Autodesk Inventor part; units mm, degrees
ref_plane "YZ Plane" through (0, 0, 0) normal (1, 0, 0) x (0, 1, 0)
ref_plane "XZ Plane" through (0, 0, 0) normal (0, 1, 0) x (-1, 0, 0)
ref_plane "XY Plane" through (0, 0, 0) normal (0, 0, 1) x (1, 0, 0)
sketch "Sketch1" plane through (0, 0, 0) normal (0, 1, 0) x (-1, 0, 0)
  line L0 (0, 0) -> (90, 0)
  line L1 (90, 0) -> (90, -50)
  line L2 (90, -50) -> (0, -50)
  line L3 (0, -50) -> (0, 0)
  line L4 (0, 0) -> (0, -16.6667)
  line L5 (0, -16.6667) -> (6, -16.6667)
  dimension "d0" = 90
  dimension "d1" = 50
  dimension "d2" = 16.6667
  dimension "d3" = 6
extrude "Extrusion1" add sketch "Sketch1" along normal blind 6
sketch "Sketch3" plane through (0, 6, 0) normal (0, 1, 0) x (1, 0, 0)
  circle A0 centre (-13, 12.5) radius 2.75
  line L0 (0, 0) -> (0, 50)
  line L1 (-90, 0) -> (0, 0)
  circle A1 centre (-13, 37.5) radius 2.75
  line L2 (-13, 12.5) -> (-18, 12.5)
  line L3 (-23, 12.5) -> (-13, 12.5) construction
  line L4 (-23, 9.75) -> (-13, 9.75)
  line L5 (-13, 15.25) -> (-23, 15.25)
  arc A2 (-23, 15.25) -> (-23, 9.75) centre (-23, 12.5) ccw
  arc A3 (-13, 9.75) -> (-13, 15.25) centre (-13, 12.5) ccw
  line L6 (-13, 37.5) -> (-18, 37.5)
  line L7 (-13, 37.5) -> (-8, 37.5) construction
  line L8 (-23, 37.5) -> (-13, 37.5) construction
  line L9 (-23, 34.75) -> (-13, 34.75)
  line L10 (-13, 40.25) -> (-23, 40.25)
  arc A4 (-23, 40.25) -> (-23, 34.75) centre (-23, 37.5) ccw
  arc A5 (-13, 34.75) -> (-13, 40.25) centre (-13, 37.5) ccw
  dimension "d21" = 5.5
  dimension "d22" = 13
  dimension "d23" = 12.5
  dimension "d26" = 25
  dimension "d87" = 5
  dimension "d88" = 5
  dimension "d89" = 180
extrude "Extrusion3" cut sketch "Sketch3" against normal through all
sketch "Sketch4" plane through (0, 6, 0) normal (0, 1, 0) x (1, 0, 0)
  arc A0 (-13, 9.75) -> (-13, 15.25) centre (-13, 12.5) ccw
  line L0 (-13, 12.5) -> (-68, 12.5)
  line L1 (-68, 12.5) -> (-74, 12.5) construction
  line L2 (-68, 15.25) -> (-74, 15.25)
  line L3 (-74, 9.75) -> (-68, 9.75)
  arc A1 (-68, 9.75) -> (-68, 15.25) centre (-68, 12.5) ccw
  arc A2 (-74, 15.25) -> (-74, 9.75) centre (-74, 12.5) ccw
  point P0 (0, 0)
  point P1 (-71, 12.5)
  dimension "d33" = 55
  dimension "d34" = 6
  dimension "d35" = 5.5
extrude "Extrusion4" cut sketch "Sketch4" against normal through all
pattern_linear "Rectangular Pattern2" count 2 spacing 25 along (0, 0, -1) of "Extrusion4"
fillet "Fillet2" radius 5 3 edges at (-90, 3, 0) (0, 3, 0) (0, 3, -50)
sketch "Sketch7" plane through (0, 6, 0) normal (0, 1, 0) x (1, 0, 0)
  arc A0 (-13, 9.75) -> (-13, 15.25) centre (-13, 12.5) ccw
  line L0 (-13, 12.5) -> (-35, 12.5)
  line L1 (-35, 12.5) -> (-55, 12.5)
  circle A1 centre (-55, 12.5) radius 2.75
  circle A2 centre (-35, 12.5) radius 2.75
  line L2 (0, 5) -> (0, 45)
  line L3 (0, 0) -> (0, 45)
  circle A3 centre (-35, 37.5) radius 2.75
  circle A4 centre (-55, 37.5) radius 2.75
  dimension "d55" = 22
  dimension "d56" = 20
  dimension "d57" = 5.5
  dimension "d58" = 5.5
  dimension "d61" = 25
extrude "Extrusion7" cut sketch "Sketch7" against normal through all
sketch "Sketch9" plane through (0, 6, 0) normal (0, 1, 0) x (1, 0, 0)
  point P0 (0, 0)
fillet "Fillet3" radius 6 1 edges at (-90, 3, -50)
properties part number "X_Carriage_Plate"
Source: CAD feature listing. Evaluate the final solid. Frame: model axes, mm. A direction names the side the tool comes from. Give positions to 0.01 mm unless a question says otherwise; leave off trailing zeros. Order: outer loops, then holes, each group sorted by start corner. A loop starts at its lowest first (then second) coordinate and runs counter-clockwise, first axis right, second up. Notation, with made-up numbers: (36.5, 73) -> (56.5, 73) arc R25 cw to (56.5, 112) -> close; hole circle Ø4 at (12, 28). An arc over 180 degrees is marked (long way). Use a Markdown table: item, result.
1) Section query C-C, the plane x = -15. Return the cut outline in (y, z), then the cut area to 3 significant figures.
Answer list:
| item | result |
|---|---|
| outline | (0, -50) -> (6, -50) -> (6, -40.25) -> (0, -40.25) -> close; (0, -34.75) -> (6, -34.75) -> (6, -15.25) -> (0, -15.25) -> close; (0, -9.75) -> (6, -9.75) -> (6, 0) -> (0, 0) -> close |
| area | 234 mm² |
2) Ray query, line 1 along Z through (x, y) = (-74, 0.45); line 2 along X through (y, z) = (3.6, -12.5); line 3 along Z through (x, y) = (-24.5, 3.95). Return the intervals inside material, ascending. Write a range as [from, to].
Answer list:
| item | result |
|---|---|
| line 1 | [-50, -40.25], [-34.75, -15.25], [-9.75, 0] |
| line 2 | [-90, -76.75], [-65.25, -57.75], [-52.25, -37.75], [-32.25, -25.75], [-10.25, 0] |
| line 3 | [-50, -39.8], [-35.2, -14.8], [-10.2, 0] |
3) Section query A-A, the plane z = -37.5. Return the cut outline in (x, y).
Answer list:
| item | result |
|---|---|
| outline | (-90, 0) -> (-76.75, 0) -> (-76.75, 6) -> (-90, 6) -> close; (-65.25, 0) -> (-57.75, 0) -> (-57.75, 6) -> (-65.25, 6) -> close; (-52.25, 0) -> (-37.75, 0) -> (-37.75, 6) -> (-52.25, 6) -> close; (-32.25, 0) -> (-25.75, 0) -> (-25.75, 6) -> (-32.25, 6) -> close; (-10.25, 0) -> (0, 0) -> (0, 6) -> (-10.25, 6) -> close |
4) Mould query, pull axis X, two halves, no side actions, for faces 1 (the cylindrical face through (-10.25, 3.04, -12.44)), 2 (the cylindrical face through (-2, 3, -1)), 3 (the flat face through (-18, 3, -15.25)), 4 (the flat face through (-90, 3, -24)). Classes: +X half, -X half, draft (parallel to the pull), parting line (faces both ways), or undercut.
Answer list:
| item | result |
|---|---|
| face 1 | undercut |
| face 2 | +X half |
| face 3 | undercut |
| face 4 | -X half |
5) Reachability of faces 5 (the flat face through (-44, 3, 0)), 6 (the flat face through (-18, 3, -40.25)) from +Z, -Z, +X, -X, +Y, -Y: full face, straight path, thin tool, end or side. Return the list, or none.
Answer list:
| item | result |
|---|---|
| face 5 | +Z, +X, -X, +Y, -Y |
| face 6 | +Y, -Y |
6) Section query B-B, the plane y = 1.5. Count the separate pieces of the cut face and the enclosed holes in it, then the cut area to 3 significant figures.
Answer list:
| item | result |
|---|---|
| separate pieces | 1 |
| enclosed holes | 8 |
| area | 4,110 mm² |
